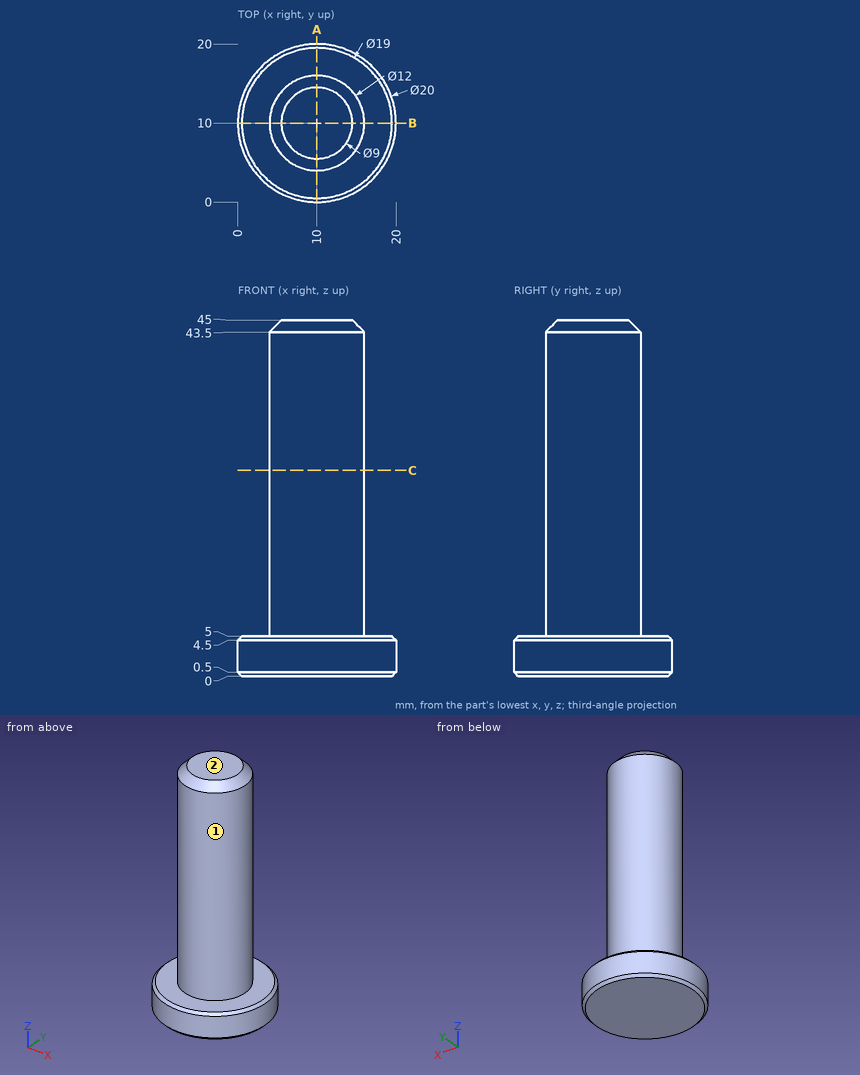
Geometry check sheet. Reference: drawing and pictorial views, mm from the part's lowest x, y, z. A direction names the side the tool comes from. Round coordinates to 2 decimals unless told otherwise and drop trailing zeros. Write each loop counter-clockwise with the first axis right and the second up, starting at its lowest first coordinate (ties: lowest second). Pieces come first, ordered by that corner, then holes. Notation, with made-up numbers: (85, 39.25) -> (91, 39.25) arc R32 cw to (91, 66.25) -> close; hole circle Ø7 at (-38.5, 66). An arc over 180 degrees is marked (long way). Answer as CSV lines item,"result". Start each with the question number.
1) Section check A-A on x = 10. Enter the section's corners in (y, z), and give its area (3 significant figures).
2) Material ranges on line 1 (Z direction, x = 8.25, y = 18.25); line 2 (Z direction, x = 4.75, y = 11.5); line 3 (X direction, y = 9, z = 15), recorded low to high. Write a range as from..to.
3) Section check C-C on z = 26. Enter the section's corners in (x, y), and give its area (3 significant figures).
4) Go/stop test with flat-tipped pins: P1, Ø10, axis at y = 11, z = 17.5, coming from the +X side; P2, Ø3, axis at x = 17, y = 6.5, coming from the +Z side; P3, Ø5, axis at y = 5.5, z = 20, coming from the -X side. Record where each tip stops, or that it passes through.
5) Tool access check on the marked faces 1 and 2. Record the directions out of +Z, -Z, +X, -X, +Y, -Y that give a thin tool (end or side, any length) a straight path to the whole face; none if there is none.
Found:
1,outline,"(0, 0.5) -> (0.5, 0) -> (19.5, 0) -> (20, 0.5) -> (20, 4.5) -> (19.5, 5) -> (16, 5) -> (16, 43.5) -> (14.5, 45) -> (5.5, 45) -> (4, 43.5) -> (4, 5) -> (0.5, 5) -> (0, 4.5) -> close"
1,area,"577 mm^2"
2,line 1,"z = 0..5"
2,line 2,"z = 0..44.04"
2,line 3,"x = 4.08..15.92"
3,outline,"circle Ø12 at (10, 10)"
3,area,"113 mm^2"
4,P1,"stops at x = 16"
4,P2,"stops at z = 5"
4,P3,"stops at x = 4.34"
5,face 1,"+Z"
5,face 2,"+Z, +X, -X, +Y, -Y"
